Can you work these out from the model? Positions are in its coordinate system, mm. A direction names the side the tool comes from. Give positions to 0.01 mm unless a question says otherwise; leave off trailing zeros. Order: outer loops, then holes, each group sorted by start corner. A loop starts at its lowest first (then second) coordinate and runs counter-clockwise, first axis right, second up. Notation, with made-up numbers: (39, 39) -> (62, 39) arc R13 cw to (62, 62) -> close; hole circle Ø4 at (-36.5, 25.5). An arc over 180 degrees is marked (long way). Answer as a JSON object with one key per item and string values.
Autodesk Inventor part; units mm, degrees
ref_plane "body1_right_XY" through (0, 0, 5.5499) normal (0, 0, -1) x (1, 0, 0)
ref_plane "body1_right_YZ" through (0, 0, 5.5499) normal (1, 0, 0) x (0, -1, 0)
ref_plane "body1_right_ZX" through (0, 0, 5.5499) normal (0, -1, 0) x (0, 0, -1)
sketch "Sketch_1" plane through (0, 0, 0) normal (0, 0, 1) x (1, 0, 0)
  line L0 (-4.4958, -2.3876) -> (-4.3434, -2.54)
  line L1 (-4.3434, -2.54) -> (4.3434, -2.54)
  line L2 (4.3434, -2.54) -> (4.4958, -2.3876)
  line L3 (4.4958, -2.3876) -> (4.4958, 2.3876)
  line L4 (4.4958, 2.3876) -> (4.3434, 2.54)
  line L5 (4.3434, 2.54) -> (-4.3434, 2.54)
  line L6 (-4.3434, 2.54) -> (-4.4958, 2.3876)
  line L7 (-4.4958, 2.3876) -> (-4.4958, -2.3876)
extrude "Extrusion1" add sketch "Sketch_1" along normal blind 5.5499
sketch "Sketch_2" plane through (0, 0, 0) normal (0, 0, 1) x (1, 0, 0)
  line L0 (-3.8862, 2.54) -> (-3.8862, -2.54)
  line L1 (-3.8862, -2.54) -> (3.8862, -2.54)
  line L2 (3.8862, -2.54) -> (3.8862, 2.54)
  line L3 (3.8862, 2.54) -> (-3.8862, 2.54)
extrude "Extrusion2" cut sketch "Sketch_2" along normal blind 0.7874
sketch "Sketch_14" plane through (0, 0, 0.7874) normal (0, 0, 1) x (1, 0, 0)
  line L0 (-3.8862, 2.413) -> (-3.8862, -2.413)
  line L1 (-3.8862, -2.413) -> (3.8862, -2.413)
  line L2 (3.8862, -2.413) -> (3.8862, 2.413)
  line L3 (3.8862, 2.413) -> (-3.8862, 2.413)
extrude "Extrusion3" cut sketch "Sketch_14" along normal blind 0.0254
sketch "Sketch_3" plane through (4.4958, 0, 0) normal (1, 0, 0) x (0, 0, -1)
  line L0 (-0.7874, 1.5494) -> (-0.7874, -1.5494)
  line L1 (-0.7874, -1.5494) -> (0, -1.9304)
  line L2 (0, -1.9304) -> (0, 1.9304)
  line L3 (0, 1.9304) -> (-0.7874, 1.5494)
extrude "Extrusion4" cut sketch "Sketch_3" against normal blind 8.9916
sketch "Sketch_4" plane through (0, 0, 4.9403) normal (0, 0, 1) x (1, 0, 0)
  line L0 (3.8862, 2.54) -> (3.8862, -2.54)
  line L1 (3.8862, -2.54) -> (4.4958, -2.54)
  line L2 (4.4958, -2.54) -> (4.4958, 2.54)
  line L3 (4.4958, 2.54) -> (3.8862, 2.54)
extrude "Extrusion5" cut sketch "Sketch_4" along normal blind 0.6096
sketch "Sketch_5" plane through (0, 0, 4.9403) normal (0, 0, 1) x (1, 0, 0)
  line L0 (-4.4958, 2.54) -> (-4.4958, -2.54)
  line L1 (-4.4958, -2.54) -> (-3.8862, -2.54)
  line L2 (-3.8862, -2.54) -> (-3.8862, 2.54)
  line L3 (-3.8862, 2.54) -> (-4.4958, 2.54)
extrude "Extrusion6" cut sketch "Sketch_5" along normal blind 0.6096
sketch "Sketch_6" plane through (0, 0, 4.9403) normal (0, 0, 1) x (1, 0, 0)
  line L0 (4.4958, 0) -> (4.9022, 0.381)
  line L1 (4.9022, 0.381) -> (4.9022, 1.524)
  line L2 (4.9022, 1.524) -> (4.4958, 1.524)
  line L3 (4.4958, 1.524) -> (4.4958, 0)
extrude "Extrusion7" add sketch "Sketch_6" against normal blind 2.032
sketch "Sketch_7" plane through (0, 0, 4.9403) normal (0, 0, 1) x (1, 0, 0)
  line L0 (-4.9022, 0.381) -> (-4.4958, 0)
  line L1 (-4.4958, 0) -> (-4.4958, 1.524)
  line L2 (-4.4958, 1.524) -> (-4.9022, 1.524)
  line L3 (-4.9022, 1.524) -> (-4.9022, 0.381)
extrude "Extrusion8" add sketch "Sketch_7" against normal blind 2.032
sketch "Sketch_8" plane through (0, 0, 4.9403) normal (0, 0, 1) x (1, 0, 0)
  line L0 (0, 2.8448) -> (0, 2.54)
  line L1 (0, 2.54) -> (1.524, 2.54)
  line L2 (1.524, 2.54) -> (1.143, 2.8448)
  line L3 (1.143, 2.8448) -> (0, 2.8448)
extrude "Extrusion9" add sketch "Sketch_8" against normal blind 2.032
ref_plane "body1_right_XY" through (0, 0, 5.5499) normal (0, 0, -1) x (1, 0, 0)
ref_plane "body1_right_YZ" through (0, 0, 5.5499) normal (1, 0, 0) x (0, -1, 0)
ref_plane "body1_right_ZX" through (0, 0, 5.5499) normal (0, -1, 0) x (0, 0, -1)
ref_plane "cp_bracker_right_XY" through (0, -2.54, 4.9403) normal (0, 1, 0) x (1, 0, 0)
ref_plane "cp_bracker_right_YZ" through (0, -2.54, 4.9403) normal (1, 0, 0) x (0, 0, -1)
ref_plane "cp_bracker_right_ZX" through (0, -2.54, 4.9403) normal (0, 0, -1) x (0, 1, 0)
ref_plane "dummy_right_XY" through (-4.4958, -2.54, 0) normal (0, 1, 0) x (1, 0, 0)
ref_plane "dummy_right_YZ" through (-4.4958, -2.54, 0) normal (1, 0, 0) x (0, 0, -1)
ref_plane "dummy_right_ZX" through (-4.4958, -2.54, 0) normal (0, 0, -1) x (0, 1, 0)
ref_plane "terminal_h_XY" through (0, 0, 0.8636) normal (0, 0, 1) x (1, 0, 0)
ref_plane "terminal_h_YZ" through (0, 0, 0.8636) normal (1, 0, 0) x (0, 1, 0)
ref_plane "terminal_h_ZX" through (0, 0, 0.8636) normal (0, 1, 0) x (0, 0, 1)
properties part number "AS11CHright12"
1. For faces 5 (the face through (-4.902, 1, 4)), 6 (the face through (4.3, 0, 4.94)), which set-ups out of +Z, -Z, +X, -X, +Y, -Y let a thin tool reach every point of the face, with its end or its side?
Worked answers:
{"face 5": "+Z, -Z, -X, +Y, -Y", "face 6": "+Z, +X, +Y, -Y"}
2. Please list where these lines run through material, in increasing order: L1, parallel to X at y = -1.85, z = 0.5; L2, parallel to Z at x = -1.5, y = -1.85; L3, parallel to Y at x = 1, z = 1.
Worked answers:
{"L1": "-4.5 to -3.89, 3.89 to 4.5", "L2": "0.81 to 5.55", "L3": "-2.54 to 2.54"}
3. If we mould it in two halves opening along Y, with no side actions, what happens to faces 1 (the face through (0, 0, 0.813)), 2 (the face through (-4.3, 0, 4.94)), 3 (the face through (0, -2.54, 3)), 4 (the face through (0.6, 2.845, 3.9))? For each: +Y half, -Y half, draft (parallel to the pull), parting line (faces both ways), or undercut.
Worked answers:
{"face 1": "undercut", "face 2": "draft", "face 3": "-Y half", "face 4": "+Y half"}
4. If we section it at C-C on x = -4: Please give me the cut outline in (y, z), then the cut area to 3 significant figures.
Worked answers:
{"outline": "(-2.54, 0) -> (-1.93, 0) -> (-1.55, 0.79) -> (1.55, 0.79) -> (1.93, 0) -> (2.54, 0) -> (2.54, 4.94) -> (-2.54, 4.94) -> close", "area": "22.4 mm²"}
5. Will these pins go through, and if not, where does the flat tip stop? pin 1 Ø1 at (x, z) = (-2.5, 1.5) entering from +Y; pin 2 Ø3 at (y, z) = (-1, 1) entering from +X; pin 3 Ø0.7 at (y, z) = (-1, 5.5) entering from -X.
Worked answers:
{"pin 1": "y = 2.54", "pin 2": "x = 4.5", "pin 3": "x = -3.89"}
6. If we section it at A-A on z = 1.8: Please give me the cut outline in (x, y), then the cut area to 3 significant figures.
Worked answers:
{"outline": "(-4.5, -2.39) -> (-4.34, -2.54) -> (4.34, -2.54) -> (4.5, -2.39) -> (4.5, 2.39) -> (4.34, 2.54) -> (-4.34, 2.54) -> (-4.5, 2.39) -> close", "area": "45.6 mm²"}
